The listing builds one solid part. Answer for the finished solid, in the listing's coordinates (mm). Face numbers are marked on the shaded views. Round coordinates to 2 decimals unless told otherwise and drop trailing zeros. Write each loop counter-clockwise with the first axis right and the second up, starting at its lowest first coordinate (ties: lowest second). Pieces come first, ordered by that corner, then holes. Notation, with made-up numbers: M 19,-29 L 70,-29 A26 cw 70,10 Z; hole C 89.5,15 d2. An arc over 180 degrees is marked long. Write each question's results on one line, items separated by ' | '.
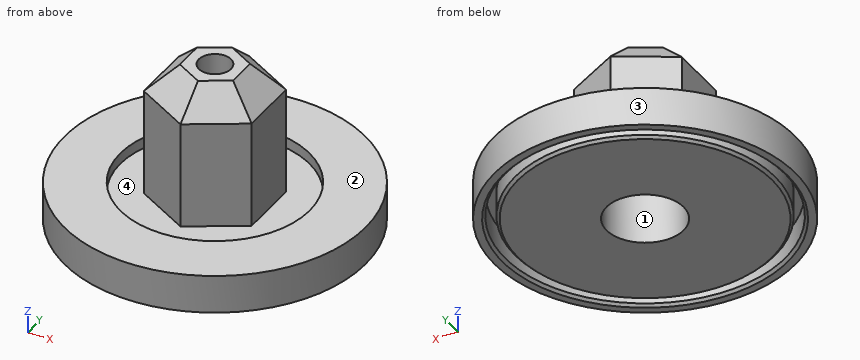
from build123d import *

# Parameters (mm, degrees)
SKETCH1_R           = 27.5
BOSS_EXTRUDE1_DEPTH = 7
SKETCH2_R           = 17.3
CUT_EXTRUDE1_DEPTH  = 2
BOSS_EXTRUDE2_DEPTH = 19.5
BOSS_EXTRUDE3_DEPTH = 5
BOSS_EXTRUDE3_TAPER = 45
SKETCH5_R           = 7.05
CUT_EXTRUDE2_DEPTH  = 16.5
SKETCH6_R           = 2.95
CUT_EXTRUDE3_DEPTH  = 43.246301613
SKETCH7_R           = 25.55
SKETCH7_R_2         = 23.75
CUT_EXTRUDE4_DEPTH  = 5
CHAMFER1_SIZE       = 0.5


with BuildPart() as part:
    # Sketch1 → Boss-Extrude1 (new body)
    with BuildSketch(Plane.XY):
        Circle(SKETCH1_R)
    extrude(amount=BOSS_EXTRUDE1_DEPTH)

    # Sketch2 → Cut-Extrude1 (cut)
    with BuildSketch(Plane.XY.offset(7)):
        Circle(SKETCH2_R)
    extrude(amount=-CUT_EXTRUDE1_DEPTH, mode=Mode.SUBTRACT)

    # Sketch3 → Boss-Extrude2 (add)
    with BuildSketch(Plane.XY.offset(5)):
        Polygon((0, 11.373800303), (-9.85, 5.686900152), (-9.85, -5.686900152), (0, -11.373800303), (9.85, -5.686900152), (9.85, 5.686900152), align=None)
    extrude(amount=BOSS_EXTRUDE2_DEPTH)

    # Sketch4 → Boss-Extrude3 (add)
    with BuildSketch(Plane.XY.offset(24.5)):
        Polygon((9.85, 5.686900152), (0, 11.373800303), (-9.85, 5.686900152), (-9.85, -5.686900152), (0, -11.373800303), (9.85, -5.686900152), align=None)
    extrude(amount=BOSS_EXTRUDE3_DEPTH, taper=BOSS_EXTRUDE3_TAPER)

    # Sketch5 → Cut-Extrude2 (cut)
    with BuildSketch(Plane(origin=(0, 0, 0), x_dir=(-1, 0, 0), z_dir=(0, 0, -1))):
        Circle(SKETCH5_R)
    extrude(amount=-CUT_EXTRUDE2_DEPTH, mode=Mode.SUBTRACT)

    # Sketch6 → Cut-Extrude3 (cut, through all)
    with BuildSketch(Plane(origin=(0, 0, 16.5), x_dir=(-1, 0, 0), z_dir=(0, 0, -1))):
        Circle(SKETCH6_R)
    extrude(amount=-CUT_EXTRUDE3_DEPTH, mode=Mode.SUBTRACT)

    # Sketch7 → Cut-Extrude4 (cut)
    with BuildSketch(Plane(origin=(0, 0, 0), x_dir=(-1, 0, 0), z_dir=(0, 0, -1))):
        Circle(SKETCH7_R)
        Circle(SKETCH7_R_2, mode=Mode.SUBTRACT)
    extrude(amount=-CUT_EXTRUDE4_DEPTH, mode=Mode.SUBTRACT)

    # Chamfer1
    chamfer1_edges = [part.edges().sort_by_distance(p)[0] for p in [
        (25.55, 0, 0),
        (23.75, 0, 0),
    ]]
    chamfer(chamfer1_edges, length=CHAMFER1_SIZE)


solid = part.part
1) Section D-D (z = 9.5) is taken. Determine the outline of the cut face in (x, y).
Return value:
outline: M -9.85,-5.69 L 0,-11.37 L 9.85,-5.69 L 9.85,5.69 L 0,11.37 L -9.85,5.69 Z; hole C 0,0 d14.1
2) Section A-A (z = 19.75) is taken. Determine the outline of the cut face in (x, y), then the cut area to 3 significant figures.
Return value:
outline: M -9.85,-5.69 L 0,-11.37 L 9.85,-5.69 L 9.85,5.69 L 0,11.37 L -9.85,5.69 Z; hole C 0,0 d5.9 | area: 309 mm²
3) Section C-C (z = 2.5) is taken. Determine the outline of the cut face in (x, y).
Return value:
outline: C 0,0 d55; C 0,0 d47.5; hole C 0,0 d51.1; hole C 0,0 d14.1
4) Find the intervals of material crossed by line 1 (Y direction, x = 0, z = 6.5); line 2 (X direction, y = -4, z = 5.5); line 3 (Y direction, x = 20, z = 2), in increasing order.
Return value:
line 1: -27.5 to -17.3, -11.37 to -7.05, 7.05 to 11.37, 17.3 to 27.5 | line 2: -27.21 to -16.83, -9.85 to -5.81, 5.81 to 9.85, 16.83 to 27.21 | line 3: -18.87 to -15.9, -12.81 to 12.81, 15.9 to 18.87
5) Each of these flat-tipped pins is pushed along its axis until it touches: pin 1 (6 mm diameter, centred on y = -12.5, z = 24.5, fed in from -X); pin 2 (16.5 mm diameter, centred on x = 7.5, y = 13, fed in from +Z); pin 3 (3 mm diameter, centred on y = -8.5, z = 21.5, fed in from +X). Where does it stop, or does it pass through?
Return value:
pin 1: x = -3.25 | pin 2: z = 27.59 | pin 3: x = 7.58
6) The mould has two halves that part along Y. Classify the marked faces 1, 2, 3 and 4: +Y half, -Y half, draft (parallel to the pull), parting line (faces both ways), or undercut.
Return value:
face 1: undercut | face 2: draft | face 3: parting line | face 4: undercut
